Check sheet for the modelled part. Datum: model origin and axes. Units: mm. Give positions to 0.01 mm unless a question says otherwise; leave off trailing zeros. Order: outer loops, then holes, each group sorted by start corner. A loop starts at its lowest first (then second) coordinate and runs counter-clockwise, first axis right, second up. Notation, with made-up numbers: (-9.75, -22.75) -> (43.25, -22.75) arc R23 ccw to (43.25, 15.25) -> close; hole circle Ø10 at (50, 0.25). An arc over 180 degrees is marked (long way). One line per question, with ' | ' between items.
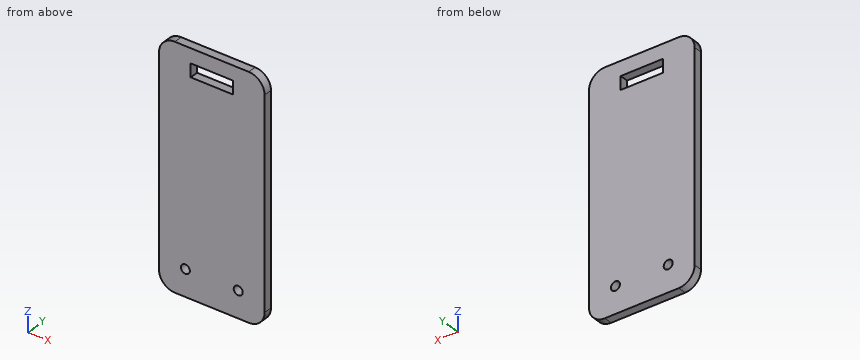
Autodesk Inventor part; units mm, degrees
ref_plane "YZ Plane" through (0, 0, 0) normal (1, 0, 0) x (0, 1, 0)
ref_plane "XZ Plane" through (0, 0, 0) normal (0, 1, 0) x (-1, 0, 0)
ref_plane "XY Plane" through (0, 0, 0) normal (0, 0, 1) x (1, 0, 0)
sketch "Sketch1" plane through (0, 0, 0) normal (0, 1, 0) x (-1, 0, 0)
  line L0 (20, 45) -> (-20, 45)
  line L1 (-20, 45) -> (-20, -45)
  line L2 (-20, -45) -> (20, -45)
  line L3 (20, -45) -> (20, 45)
  line L4 (20, 45) -> (-20, -45) construction
  line L5 (-20, 45) -> (20, -45) construction
  point P0 (0, 0)
  dimension "d0" = 40
  dimension "d1" = 90
extrude "Plate1" add sketch "Sketch1" along normal blind 3.2
sketch "Sketch2" plane through (0, 3.2, 0) normal (0, 1, 0) x (1, 0, 0)
  line L0 (-20, -45) -> (20, -45)
  line L1 (0, -45) -> (0, 35)
  line L2 (0, 35) -> (-10, 35)
  point P0 (0, 0)
  point P1 (10, 35)
  point P2 (10, 35)
  dimension "d3" = 80
  dimension "d4" = 10
hole "Hole1" at (-10, 3.2, -35) at (10, 3.2, -35) direction (0, -1, 0) diameter 3.4 depth 3.2 tip angle 118
sketch "Sketch4" plane through (0, 0, 0) normal (0, -1, 0) x (1, 0, 0)
  line L0 (8, 39.559) -> (-8, 39.559)
  line L1 (-8, 39.559) -> (-8, 34.559)
  line L2 (-8, 34.559) -> (8, 34.559)
  line L3 (8, 34.559) -> (8, 39.559)
  line L4 (8, 39.559) -> (-8, 34.559) construction
  line L5 (-8, 39.559) -> (8, 34.559) construction
  line L6 (-20, 45) -> (20, 45)
  point P0 (0, 0)
  point P1 (0, 37.059)
  dimension "d12" = 16
  dimension "d13" = 5
  dimension "d17" = 7.941
extrude "Cut1" cut sketch "Sketch4" against normal blind 3.2
fillet "Corner Round1" radius 6 4 edges at (20, 1.6, 45) (-20, 1.6, 45) (20, 1.6, -45) (-20, 1.6, -45)
equation "\"d10\" = Thickness"
equation "\"d14\" = Thickness"
equation "\"d2\" = Thickness"
equation "\"BendReliefWidth\" = Thickness"
equation "\"BendReliefDepth\" = 0.5 * Thickness"
equation "\"CornerReliefSize\" = 4 * Thickness"
equation "\"MinimumRemnant\" = 2 * Thickness"
equation "\"TransitionRadius\" = BendRadius"
equation "\"JacobiRadiusSize\" = BendRadius"
equation "\"GapSize\" = Thickness"
properties part number "SP40V1 Chapa Base"
Q1. Section check B-B (z = -35). Enter the section's corners in (x, y).
Result sheet:
outline: (-20, 0) -> (-11.7, 0) -> (-11.7, 3.2) -> (-20, 3.2) -> close; (-8.3, 0) -> (8.3, 0) -> (8.3, 3.2) -> (-8.3, 3.2) -> close; (11.7, 0) -> (20, 0) -> (20, 3.2) -> (11.7, 3.2) -> close
Q2. Thickness scan on line 1 (X direction, y = 1.8, z = -35); line 2 (Z direction, x = 7, y = 1.1); line 3 (Z direction, x = -10, y = 2.25). Record the ranges inside material, lowest first.
Result sheet:
line 1: x = -20 to -11.7, -8.3 to 8.3, 11.7 to 20 | line 2: z = -45 to 34.56, 39.56 to 45 | line 3: z = -45 to -36.7, -33.3 to 45
Q3. Section check D-D (x = -5.5). Enter the section's corners in (y, z), and give its area (3 significant figures).
Result sheet:
outline: (0, -45) -> (3.2, -45) -> (3.2, 34.56) -> (0, 34.56) -> close; (0, 39.56) -> (3.2, 39.56) -> (3.2, 45) -> (0, 45) -> close | area: 272 mm2
Q4. Section check C-C (y = 2.7). Enter the section's corners in (x, z), and give its area (3 significant figures).
Result sheet:
outline: (-20, -39) arc R6 ccw to (-14, -45) -> (14, -45) arc R6 ccw to (20, -39) -> (20, 39) arc R6 ccw to (14, 45) -> (-14, 45) arc R6 ccw to (-20, 39) -> close; hole circle Ø3.4 at (-10, -35); hole (-8, 34.56) -> (8, 34.56) -> (8, 39.56) -> (-8, 39.56) -> close; hole circle Ø3.4 at (10, -35) | area: 3,470 mm2
Q5. Depth check by flat-ended pin: pin 1 Ø5 at (x, z) = (4, -2) entering from -Y; pin 2 Ø1.5 at (x, y) = (-15, 1.5) entering from +Z. Enter the tip coordinate at first touch or a pass-through.
Result sheet:
pin 1: stops at y = 0 | pin 2: stops at z = 44.99
Q6. Section check A-A (x = 10). Enter the section's corners in (y, z), and give its area (3 significant figures).
Result sheet:
outline: (0, -45) -> (3.2, -45) -> (3.2, -36.7) -> (0, -36.7) -> close; (0, -33.3) -> (3.2, -33.3) -> (3.2, 45) -> (0, 45) -> close | area: 277 mm2
